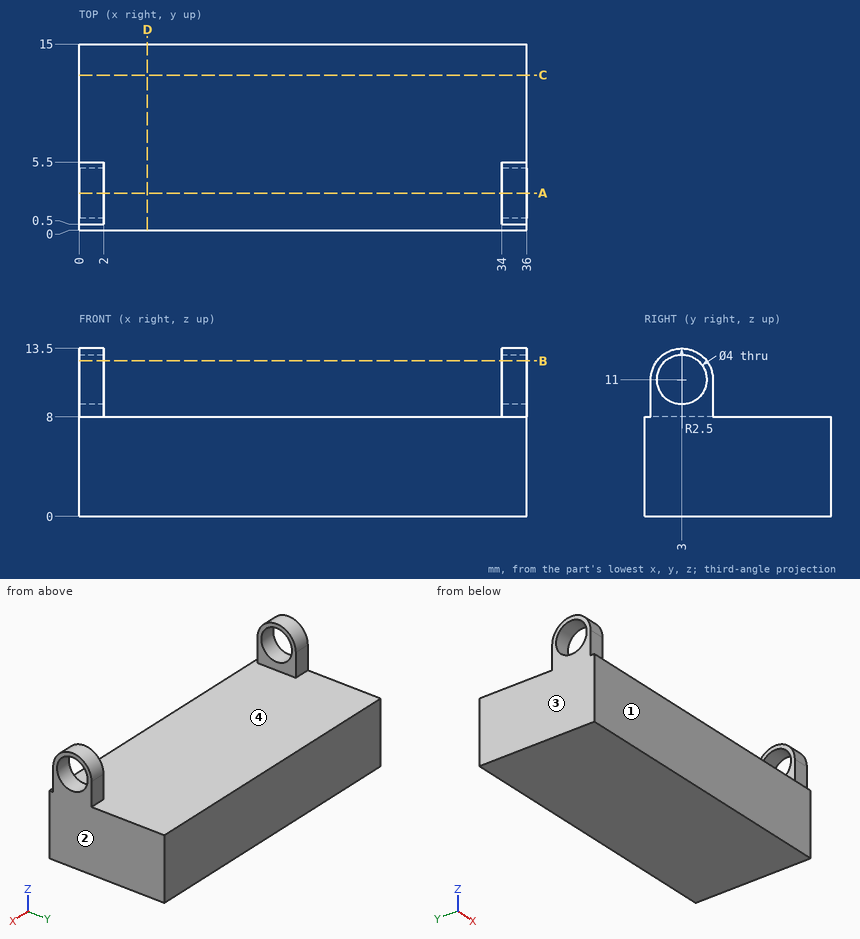
Check sheet for the drawn part. Datum: minimum x, y, z corner. Units: mm. Round coordinates to 2 decimals unless told otherwise and drop trailing zeros. Loops run counter-clockwise (first coordinate to the right, second up) from the corner with the lowest first, then second, coordinate; pieces in that order, holes last.
Item 1: Cross-section at B-B on z = 12.5. Record the boundary of the cut face in (x, y).
Item 2: Cross-section at A-A on y = 3. Record the boundary of the cut face in (x, z).
Item 3: Cross-section at C-C on y = 12.5. Record the boundary of the cut face in (x, z), then the cut area to 3 significant figures.
Item 4: Gauge pin test, flat ends, axial feed: pin 1 (0.6 mm diameter, centred on x = 35.5, z = 9.5, fed in from +Y); pin 2 (3 mm diameter, centred on x = 12.5, y = 3.5, fed in from +Z); pin 3 (1 mm diameter, centred on x = 1, z = 10, fed in from -Y). Record the tip position at first contact, or that the pin passes through.
Item 5: Thickness scan on line 1 (X direction, y = 2, z = 8.75); line 2 (Y direction, x = 0.65, z = 11); line 3 (Z direction, x = 8, y = 6.5). Record the ranges inside material, lowest first.
Item 6: Mould release check, pull along X, two halves, no side actions. Record for the marked faces 1, 2, 3 and 4: pulls with the +X half, pulls with the -X half, needs draft (parallel to the pull), parting line crosses it, or undercut.
Item 7: Cross-section at D-D on x = 5.5. Record the boundary of the cut face in (y, z), then the cut area to 3 significant figures.
Answer sheet:
1. outline: (0, 1) - (2, 1) - (2, 1.68) - (0, 1.68) - close; (0, 4.32) - (2, 4.32) - (2, 5) - (0, 5) - close; (34, 1) - (36, 1) - (36, 1.68) - (34, 1.68) - close; (34, 4.32) - (36, 4.32) - (36, 5) - (34, 5) - close
2. outline: (0, 0) - (36, 0) - (36, 9) - (34, 9) - (34, 8) - (2, 8) - (2, 9) - (0, 9) - close; (0, 13) - (2, 13) - (2, 13.5) - (0, 13.5) - close; (34, 13) - (36, 13) - (36, 13.5) - (34, 13.5) - close
3. outline: (0, 0) - (36, 0) - (36, 8) - (0, 8) - close
3. area: 288 mm2
4. pin 1: stops at y = 5.5
4. pin 2: stops at z = 8
4. pin 3: stops at y = 0.5
5. line 1: x = 0 to 2, 34 to 36
5. line 2: y = 0.5 to 1, 5 to 5.5
5. line 3: z = 0 to 8
6. face 1: needs draft
6. face 2: pulls with the +X half
6. face 3: pulls with the -X half
6. face 4: undercut
7. outline: (0, 0) - (15, 0) - (15, 8) - (0, 8) - close
7. area: 120 mm2
